For this review, take the finished solid that the model builds, in its own axes (mm). A direction names the side the tool comes from. Coordinates: 2 decimals unless noted, no trailing zeros. Write each loop counter-clockwise with the first axis right and the second up, starting at its lowest first coordinate (ties: lowest second). Pieces come first, ordered by that corner, then holes.
1) We need section D-D on x = -12.7. Write out the cut boundary in (y, z), then the cut area to 4 significant figures.
2) We need section B-B on x = 20. Write out the cut boundary in (y, z), then the cut area to 3 significant figures.
3) We need section C-C on y = 2.5. Write out the cut boundary in (x, z).
4) Mouldability with a two-part tool opening along Y and no side actions: class faces 4 (the face through (-8.8, 5.2, 1.5)), 5 (the face through (0, -8, 14)), 6 (the face through (-18.5, -9.97, 13.07)), 7 (the face through (9.486, 0.154, 1.479)) as pulls with the +Y half, pulls with the -Y half, needs draft (parallel to the pull), parting line crosses it, or undercut.
5) To check wall thickness, follow line 1 along Z through (x, y) = (20, -10.85); line 2 along Y through (x, z) = (2, 2); line 3 along Y through (x, z) = (-5.5, 11.75). State the ranges of each line that lie inside material, in increasing order.
6) For faces 1 (the face through (0, -7, 3)), 2 (the face through (0, -7, 0)), 3 (the face through (-9.64, -5.18, 1.48)), list the 3-axis set-ups (+Z, -Z, +X, -X, +Y, -Y) from which the entire face can be reached by the end or side of a thin tool; tool diameter is ignored.
7) Insertion check: P1, Ø8, axis at y = -2, z = 13.5, coming from the +X side; P2, Ø3, axis at x = -14, y = -5.5, coming from the +Z side; P3, Ø4, axis at x = -0.5, z = 16, coming from the +Y side. Each pin has a flat end and moves straight along its axis. Give the tip position at first contact, or say it passes through.
8) We need section A-A on z = 13. Write out the cut boundary in (x, y).
from build123d import *

# Parameters (mm, degrees)
F0_W     = 50
F0_H     = 15
F0_R     = 1.25
F1_DEPTH = 3
F0_H_2   = 4
F2_DEPTH = 25
F4_R     = 1.5
F5_DEPTH = 4.001


with BuildPart() as f1:
    # F0 (on Top) → F1 (new body)
    with BuildSketch(Plane.XY):
        with Locations((0, -0.5)):
            Rectangle(F0_W, F0_H)
        with Locations((-12.7, 0)):
            Circle(F0_R, mode=Mode.SUBTRACT)
        with BuildLine():
            ThreePointArc((-9.0826785685, 4.590535746), (-8.7611236503, 5.2384225572), (-8.0867853621, 5.5))
            Line((-8.0867853621, 5.5), (8.0867853621, 5.5))
            ThreePointArc((8.0867853621, 5.5), (8.7611236503, 5.2384225572), (9.0826785685, 4.590535746))
            Line((9.0826785685, 4.590535746), (9.9008603867, -4.409464254))
            ThreePointArc((9.9008603867, -4.409464254), (9.6433897375, -5.1743382882), (8.9049671803, -5.5))
            Line((8.9049671803, -5.5), (-8.9049671803, -5.5))
            ThreePointArc((-8.9049671803, -5.5), (-9.6433897375, -5.1743382882), (-9.9008603867, -4.409464254))
            Line((-9.9008603867, -4.409464254), (-9.0826785685, 4.590535746))
        make_face(mode=Mode.SUBTRACT)
        with Locations((12.7, 0)):
            Circle(F0_R, mode=Mode.SUBTRACT)
    extrude(amount=F1_DEPTH)

    # F0 (on Top) → F2 (join)
    with BuildSketch(Plane.XY):
        with Locations((0, -10)):
            Rectangle(F0_W, F0_H_2)
    extrude(amount=F2_DEPTH)

    # F4 (on offset) → F5 (cut, through all)
    with BuildSketch(Plane(origin=(0, -8, 0), x_dir=(-1, 0, 0), z_dir=(0, 1, 0))):
        with Locations((-20, 13)):
            Circle(F4_R)
        with Locations((20, 13)):
            Circle(F4_R)
    extrude(amount=-F5_DEPTH, mode=Mode.SUBTRACT)


solid = f1.part
Result:
1. outline: (-12, 0) - (-1.25, 0) - (-1.25, 3) - (-8, 3) - (-8, 25) - (-12, 25) - close; (1.25, 0) - (7, 0) - (7, 3) - (1.25, 3) - close
1. area: 137.5 mm2
2. outline: (-12, 0) - (7, 0) - (7, 3) - (-8, 3) - (-8, 11.5) - (-12, 11.5) - close; (-12, 14.5) - (-8, 14.5) - (-8, 25) - (-12, 25) - close
2. area: 133 mm2
3. outline: (-25, 0) - (-9.27, 0) - (-9.27, 3) - (-25, 3) - close; (9.27, 0) - (25, 0) - (25, 3) - (9.27, 3) - close
4. face 4: undercut
4. face 5: pulls with the +Y half
4. face 6: needs draft
4. face 7: undercut
5. line 1: z = 0 to 11.5, 14.5 to 25
5. line 2: y = -12 to -5.5, 5.5 to 7
5. line 3: y = -12 to -8
6. face 1: +Z, +X, -X, +Y
6. face 2: -Z, +X, -X, +Y, -Y
6. face 3: +Z, -Z
7. P1: passes through
7. P2: stops at z = 3
7. P3: stops at y = -8
8. outline: (-25, -12) - (-21.5, -12) - (-21.5, -8) - (-25, -8) - close; (-18.5, -12) - (18.5, -12) - (18.5, -8) - (-18.5, -8) - close; (21.5, -12) - (25, -12) - (25, -8) - (21.5, -8) - close
